```python
from build123d import *

# Parameters (mm, degrees)
BOSS_EXTRUDE1_DEPTH                 = 18
SKETCH2_W                           = 28
SKETCH2_H                           = 36
CUT_EXTRUDE1_DEPTH                  = 43
CUT_EXTRUDE2_DEPTH                  = 43
SKETCH4_W                           = 20
SKETCH4_H                           = 20
CUT_EXTRUDE3_DEPTH                  = 8
FILLET1_R                           = 6
CUT_EXTRUDE4_DEPTH                  = 12.0000001
F_6_0MM_DOWEL_HOLE3_D               = 6
F_6_0MM_DOWEL_HOLE3_DEPTH           = 6
F_6_0MM_DOWEL_HOLE3_TIP             = 1.802581857
F_6_0MM_DOWEL_HOLE3_ON_FACE_2_D     = 6
F_6_0MM_DOWEL_HOLE3_ON_FACE_2_DEPTH = 6
F_6_0MM_DOWEL_HOLE3_ON_FACE_2_TIP   = 1.802581857


with BuildPart() as part:
    # Sketch1 → Boss-Extrude1 (new body, symmetric)
    with BuildSketch(Plane.XY):
        with BuildLine():
            Line((-82, 0), (82, 0))
            Line((82, 0), (79, 11))
            Line((79, 11), (50, 11))
            Line((50, 11), (50, 54))
            Line((50, 54), (22, 54))
            Line((22, 54), (22, 41))
            Line((22, 41), (18.761663039, 41))
            ThreePointArc((18.761663039, 41), (0, 19), (-18.761663039, 41))
            Line((-18.761663039, 41), (-22, 41))
            Line((-22, 41), (-22, 54))
            Line((-22, 54), (-50, 54))
            Line((-50, 54), (-50, 11))
            Line((-50, 11), (-79, 11))
            Line((-79, 11), (-82, 0))
        make_face()
    boss_extrude1 = extrude(amount=BOSS_EXTRUDE1_DEPTH, both=True)

    # Sketch2 → Cut-Extrude1 (cut)
    with BuildSketch(Plane(origin=(0, 54, 0), x_dir=(1, 0, 0), z_dir=(0, 1, 0))):
        with Locations((-36, 0)):
            Rectangle(SKETCH2_W, SKETCH2_H)
    extrude(amount=-CUT_EXTRUDE1_DEPTH, mode=Mode.SUBTRACT)

    # Mirror1: Boss-Extrude1 across plane
    add(boss_extrude1.mirror(Plane(origin=(0, 0, 0), x_dir=(0, 0, 1), z_dir=(1, 0, 0))))

    # Sketch3 → Cut-Extrude2 (cut)
    with BuildSketch(Plane(origin=(0, 54, 0), x_dir=(1, 0, 0), z_dir=(0, 1, 0))):
        with BuildLine():
            Line((44.497190923, 18), (50, 18))
            Line((50, 18), (50, -18))
            Line((50, -18), (44.497190923, -18))
            ThreePointArc((44.497190923, -18), (48, 0), (44.497190923, 18))
        make_face()
    cut_extrude2 = extrude(amount=-CUT_EXTRUDE2_DEPTH, mode=Mode.SUBTRACT)

    # Mirror2: Cut-Extrude2 across plane
    add(cut_extrude2.mirror(Plane(origin=(0, 0, 0), x_dir=(0, 0, 1), z_dir=(1, 0, 0))), mode=Mode.SUBTRACT)

    # Sketch4 → Cut-Extrude3 (cut)
    with BuildSketch(Plane.XZ):
        with Locations((-31, 0)):
            Rectangle(SKETCH4_W, SKETCH4_H)
    cut_extrude3 = extrude(amount=-CUT_EXTRUDE3_DEPTH, mode=Mode.SUBTRACT)

    # Mirror3: Cut-Extrude3 across plane
    add(cut_extrude3.mirror(Plane(origin=(0, 0, 0), x_dir=(0, 0, 1), z_dir=(1, 0, 0))), mode=Mode.SUBTRACT)

    # Fillet1
    fillet1_edges = [part.edges().sort_by_distance(p)[0] for p in [
        (-48, 11, 0),
        (48, 11, 0),
    ]]
    fillet(fillet1_edges, radius=FILLET1_R)

    # Sketch10 → Ø6.0mm Dowel Hole2 (revolve, cut)
    with BuildSketch(Plane(origin=(-31, 54, 0), x_dir=(0, 0, 1), z_dir=(1, 0, 0))):
        Polygon((0, 0), (0, 56.703872786), (4.5, 54), (4.5, 0), align=None)
    f_6_0mm_dowel_hole2 = revolve(axis=Axis((-31, 60.35, 0), (0, -1, 0)), mode=Mode.SUBTRACT)

    # Mirror4: Ø6.0mm Dowel Hole2 across plane
    add(f_6_0mm_dowel_hole2.mirror(Plane(origin=(0, 0, 0), x_dir=(0, 0, 1), z_dir=(1, 0, 0))), mode=Mode.SUBTRACT)

    # Sketch18 → Cut-Extrude4 (cut, through all)
    with BuildSketch(Plane(origin=(0, 11, 0), x_dir=(1, 0, 0), z_dir=(0, 1, 0))):
        with BuildLine():
            Line((-67.5, 4.5), (-60.5, 4.5))
            ThreePointArc((-60.5, 4.5), (-56, 0), (-60.5, -4.5))
            Line((-60.5, -4.5), (-67.5, -4.5))
            ThreePointArc((-67.5, -4.5), (-72, 0), (-67.5, 4.5))
        make_face()
    cut_extrude4 = extrude(amount=-CUT_EXTRUDE4_DEPTH, mode=Mode.SUBTRACT)

    # Mirror5: Cut-Extrude4 across plane
    add(cut_extrude4.mirror(Plane(origin=(0, 0, 0), x_dir=(0, 0, 1), z_dir=(1, 0, 0))), mode=Mode.SUBTRACT)

    # Ø6.0mm Dowel Hole3
    with Locations(Plane(origin=(0, 19, 0), x_dir=(1, 0, 0), z_dir=(0, 1, 0))):
        with Locations((0, 0)):
            Hole(F_6_0MM_DOWEL_HOLE3_D / 2, depth=F_6_0MM_DOWEL_HOLE3_DEPTH)
            with Locations((0, 0, -(F_6_0MM_DOWEL_HOLE3_DEPTH + F_6_0MM_DOWEL_HOLE3_TIP / 2))):  # 118° drill point
                Cone(0, F_6_0MM_DOWEL_HOLE3_D / 2, F_6_0MM_DOWEL_HOLE3_TIP, mode=Mode.SUBTRACT)

    # Ø6.0mm Dowel Hole3 on face 2
    with Locations(Plane(origin=(-148.466540519, 0, -78.953744881), x_dir=(1, 0, 0), z_dir=(0, 1, 0))):
        with Locations((0, 0)):
            Hole(F_6_0MM_DOWEL_HOLE3_ON_FACE_2_D / 2, depth=F_6_0MM_DOWEL_HOLE3_ON_FACE_2_DEPTH)
            with Locations((0, 0, -(F_6_0MM_DOWEL_HOLE3_ON_FACE_2_DEPTH + F_6_0MM_DOWEL_HOLE3_ON_FACE_2_TIP / 2))):  # 118° drill point
                Cone(0, F_6_0MM_DOWEL_HOLE3_ON_FACE_2_D / 2, F_6_0MM_DOWEL_HOLE3_ON_FACE_2_TIP, mode=Mode.SUBTRACT)


solid = part.part
```
Here's how the part is built. I have some questions about the finished solid (model axes, mm). A direction names the side the tool comes from. Round coordinates to 2 decimals unless told otherwise and drop trailing zeros. Loops run counter-clockwise (first coordinate to the right, second up) from the corner with the lowest first, then second, coordinate; pieces in that order, holes last. Notation, with made-up numbers: (0, 79.5) -> (51, 79.5) arc R10 cw to (51, 86.5) -> close; hole circle Ø2 at (-30, 5). An arc over 180 degrees is marked (long way). Answer as CSV lines item,"result". Start each with the question number.
1. Imagine slicing it at A-A on y = 43. Write out the boundary of the cut face in (x, z), plus the area to 3 significant figures.
2. Imagine slicing it at B-B on x = -31. Write out the boundary of the cut face in (y, z), plus the area to 3 significant figures.
3. I'm going to push flat-ended pins straight in: P1, Ø12, axis at y = 37.5, z = -3, coming from the -X side; P2, Ø2.5, axis at x = -20.5, z = 6.5, coming from the +Y side; P3, Ø3, axis at y = 10, z = -6.5, coming from the -X side; P4, Ø16, axis at x = 33, z = 2.5, coming from the -Y side. Where does each tip first touch, or does it pass through?
4. I need wall thicknesses on probe 1 along Z at (x, y) = (0, 17.5); probe 2 along X at (y, z) = (25, 3); probe 3 along X at (y, z) = (30, 0). Which ranges of each line are inside material? Lowest first, please. Write a range as from..to.
5. For faces 5 (the face through (-0.11, 11.51, 0.51)), 6 (the face through (64, 6, 4.5)), 7 (the face through (38, 54, 0)), 8 (the face through (-21, 4, 0)), 9 (the face through (22, 48, 0)), which set-ups out of +Z, -Z, +X, -X, +Y, -Y let a thin tool reach every point of the face, with its end or its side?
6. If we mould it in two halves opening along X, with no side actions, what happens to faces 1 (the face through (56, 6, 0)), 2 (the face through (-71, 11, 4)), 3 (the face through (0, 19, 4)), 4 (the face through (-48, 36, 0))? For each: pulls with the +X half, pulls with the -X half, needs draft (parallel to the pull), parting line crosses it, or undercut.
Solution:
1,outline,"(-44.5, -18) -> (-22, -18) -> (-22, 18) -> (-44.5, 18) arc R48 ccw to start; (22, -18) -> (44.5, -18) arc R48 ccw to (44.5, 18) -> (22, 18) -> close; hole circle Ø9 at (-31, 0); hole circle Ø9 at (31, 0)"
1,area,"1,660 mm²"
2,outline,"(0, -18) -> (54, -18) -> (54, -4.5) -> (8, -4.5) -> (8, -10) -> (0, -10) -> close; (0, 10) -> (8, 10) -> (8, 4.5) -> (54, 4.5) -> (54, 18) -> (0, 18) -> close"
2,area,"1,370 mm²"
3,P1,"x = -48"
3,P2,"y = 41"
3,P3,"x = -79.68"
3,P4,"y = 0"
4,probe 1,"-18..-3, 3..18"
4,probe 2,"-47.91..-34.35, -27.65..-13.86, 13.86..27.65, 34.35..47.91"
4,probe 3,"-48..-35.5, -26.5..-17.23, 17.23..26.5, 35.5..48"
5,face 5,"+Y"
5,face 6,"+Y, -Y"
5,face 7,"+Z, -Z, +X, -X, +Y"
5,face 8,"-Y"
5,face 9,"+Z, -Z, +Y"
6,face 1,"undercut"
6,face 2,"needs draft"
6,face 3,"undercut"
6,face 4,"pulls with the -X half"
